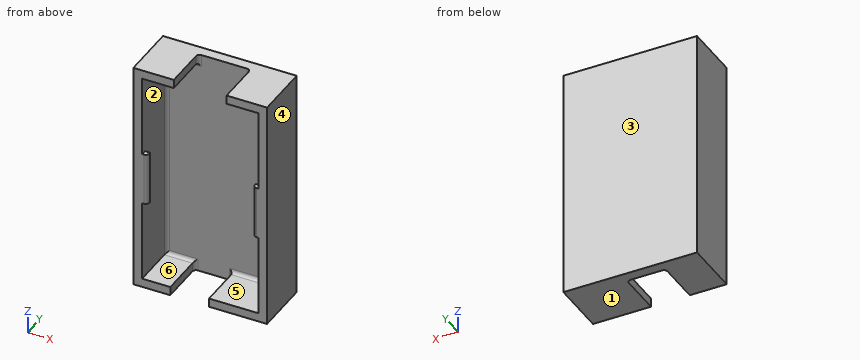
from build123d import *

# Parameters (mm, degrees)
SKETCH1_W           = 38
SKETCH1_H           = 66
BOSS_EXTRUDE1_DEPTH = 3
BOSS_EXTRUDE3_DEPTH = 13
SKETCH5_W           = 15
SKETCH5_H           = 1.5
BOSS_EXTRUDE4_DEPTH = 1.5
FILLET2_R           = 1
FILLET3_R           = 1


with BuildPart() as part:
    # Sketch1 → Boss-Extrude1 (new body)
    with BuildSketch(Plane(origin=(0, 0, 0), x_dir=(1, 0, 0), z_dir=(0, 1, 0))):
        Rectangle(SKETCH1_W, SKETCH1_H)
    extrude(amount=BOSS_EXTRUDE1_DEPTH)

    # Sketch2 → Boss-Extrude3 (add)
    with BuildSketch(Plane(origin=(0, 0, 0), x_dir=(1, 0, 0), z_dir=(0, 1, 0))):
        Polygon((2.5, 30.5), (2.5, 33), (19, 33), (19, -33), (7.5, -33), (7.5, -30.5), (16.5, -30.5), (16.5, 30.5), align=None)
        Polygon((-19, 33), (-19, -33), (-7.5, -33), (-7.5, -30.5), (-16.5, -30.5), (-16.5, 30.5), (-8.5, 30.5), (-8.5, 33), align=None)
    extrude(amount=-BOSS_EXTRUDE3_DEPTH)

    # Sketch5 → Boss-Extrude4 (add)
    with BuildSketch(Plane.ZY.offset(-16.5)):
        with Locations((0, -12.25)):
            Rectangle(SKETCH5_W, SKETCH5_H)
    boss_extrude4 = extrude(amount=BOSS_EXTRUDE4_DEPTH)

    # Mirror1: Boss-Extrude4 across plane
    add(boss_extrude4.mirror(Plane(origin=(0, 0, 0), x_dir=(0, 0, 1), z_dir=(1, 0, 0))))

    # Fillet2
    fillet2_edges = [part.edges().sort_by_distance(p)[0] for p in [
        (15, -13, 0),
        (-15, -13, 0),
    ]]
    fillet(fillet2_edges, radius=FILLET2_R)

    # Fillet3
    fillet3_edges = [part.edges().sort_by_distance(p)[0] for p in [
        (-8.5, 0, -31.75),
        (2.5, 0, -31.75),
        (-12.5, 0, -30.5),
        (9.5, 0, -30.5),
        (16.5, 0, 0),
        (7.5, 0, 31.75),
        (12, 0, 30.5),
        (-16.5, 0, 0),
        (-12, 0, 30.5),
        (-7.5, 0, 31.75),
    ]]
    fillet(fillet3_edges, radius=FILLET3_R)


solid = part.part
Design review of the part built by this model. Coordinates are the model's own, in mm. Face numbers are marked on the shaded views. A direction names the side the tool comes from. Give positions to 0.01 mm unless a question says otherwise; leave off trailing zeros. Loops run counter-clockwise (first coordinate to the right, second up) from the corner with the lowest first, then second, coordinate; pieces in that order, holes last. Notation, with made-up numbers: (-36.5, 54.5) -> (-21.5, 54.5) arc R25 ccw to (-21.5, 78.5) -> close; hole circle Ø6 at (65.5, 16). An arc over 180 degrees is marked (long way). One line per question, with ' | ' between items. Start each with the question number.
(1) We need section B-B (x = 12). State the section outline as (y, z) points.
(2) For the marked faces 1 and 2, list the 3-axis set-ups (+Z, -Z, +X, -X, +Y, -Y) from which the entire face can be reached by the end or side of a thin tool; tool diameter is ignored.
(3) We need section A-A (y = -5.5). State the section outline as (x, z) points.
(4) Draft analysis for pull direction X (two halves, no side actions). For the marked faces 3, 4, 5 and 6, state which applies: +X half, -X half, draft (parallel to the pull), parting line (faces both ways), or undercut.
(5) For line 1 (X direction, y = -1.5, z = -1.5); line 2 (Z direction, x = 9.5, y = -1.5); line 3 (Y direction, x = -9, z = 18), list the stretches that pass through material, from the lowest coordinate up.
(6) We need section D-D (z = 14.5). State the section outline as (x, y) points.
(7) We need section C-C (z = 0). State the section outline as (x, y) points, and give its area (4 significant figures).
The answers:
1) outline: (-13, -33) -> (3, -33) -> (3, 33) -> (-13, 33) -> (-13, 30.5) -> (-1, 30.5) arc R1 cw to (0, 29.5) -> (0, -29.5) arc R1 cw to (-1, -30.5) -> (-13, -30.5) -> close
2) face 1: -Z, +X, -X, +Y, -Y | face 2: none
3) outline: (-19, -33) -> (-8.5, -33) -> (-8.5, -30.5) -> (-16.5, -30.5) -> (-16.5, 30.5) -> (-7.5, 30.5) -> (-7.5, 33) -> (-19, 33) -> close; (2.5, -33) -> (19, -33) -> (19, 33) -> (7.5, 33) -> (7.5, 30.5) -> (16.5, 30.5) -> (16.5, -30.5) -> (2.5, -30.5) -> close
4) face 3: draft | face 4: +X half | face 5: undercut | face 6: undercut
5) line 1: x = -19 to -16.5, 16.5 to 19 | line 2: z = -33 to -30.5, 30.5 to 33 | line 3: y = 0 to 3
6) outline: (-19, -13) -> (-16.5, -13) -> (-16.5, -1) arc R1 cw to (-15.5, 0) -> (15.5, 0) arc R1 cw to (16.5, -1) -> (16.5, -13) -> (19, -13) -> (19, 3) -> (-19, 3) -> close
7) outline: (-19, -13) -> (-16, -13) arc R1 ccw to (-15, -12) -> (-15, -11.5) -> (-16.5, -11.5) -> (-16.5, -1) arc R1 cw to (-15.5, 0) -> (15.5, 0) arc R1 cw to (16.5, -1) -> (16.5, -11.5) -> (15, -11.5) -> (15, -12) arc R1 ccw to (16, -13) -> (19, -13) -> (19, 3) -> (-19, 3) -> close | area: 183.5 mm^2
